```python
from build123d import *

# Parameters (mm, degrees)
BOSS_EXTRUDE1_DEPTH      = 54
BOSS_EXTRUDE1_DEPTH_BACK = 54
SKETCH2_R                = 18
SKETCH3_R                = 4
CUT_EXTRUDE1_DEPTH       = 122
SKETCH4_R                = 1.5
CUT_EXTRUDE2_DEPTH       = 5


with BuildPart() as part:
    # Sketch2 → Boss-Extrude1 (new, two sides: drawn at the far end of the back side and taken through both)
    with BuildSketch(Plane.XY.offset(-BOSS_EXTRUDE1_DEPTH_BACK)):
        Circle(SKETCH2_R)
    extrude(amount=BOSS_EXTRUDE1_DEPTH + BOSS_EXTRUDE1_DEPTH_BACK)

    # Sketch3 → Cut-Extrude1 (cut)
    with BuildSketch(Plane.XY.offset(54)):
        Circle(SKETCH3_R)
    extrude(amount=-CUT_EXTRUDE1_DEPTH, mode=Mode.SUBTRACT)

    # Sketch4 → Cut-Extrude2 (cut)
    with BuildSketch(Plane(origin=(0, 0, -54), x_dir=(-1, 0, 0), z_dir=(0, 0, -1))):
        with Locations((0, 14)):
            Circle(SKETCH4_R)
        with Locations((14, 0)):
            Circle(SKETCH4_R)
        with Locations((0, -14)):
            Circle(SKETCH4_R)
        with Locations((-14, 0)):
            Circle(SKETCH4_R)
    extrude(amount=-CUT_EXTRUDE2_DEPTH, mode=Mode.SUBTRACT)


solid = part.part
```
Could you check a few things on this model? Use its own coordinates, in mm. A direction names the side the tool comes from. Coordinates: 2 decimals unless noted, no trailing zeros. Order: outer loops, then holes, each group sorted by start corner. A loop starts at its lowest first (then second) coordinate and runs counter-clockwise, first axis right, second up. Notation, with made-up numbers: M 86,19 L 140,19 A21 ccw 140,46 Z; hole C -5.75,78.25 d9. An arc over 180 degrees is marked long. Use a Markdown table: item, result. Add a question column.
Q1. I want a section at A-A on y = 0. List the corners of the cut face in (x, z) for me, then the cut area to 3 significant figures.
Q2. We'd pull the mould along X, two halves only. Please class faces 1 (the cylindrical face through (-2.343, 17.847, -0.756)), 2 (the cylindrical face through (0.325, 12.536, -51.535)), 3 (the flat face through (-4.3, 0.3, 54)): pulls with the +X half, pulls with the -X half, needs draft (parallel to the pull), parting line crosses it, or undercut.
Q3. I want a section at C-C on z = 42. List the corners of the cut face in (x, y) for me, then the cut area to 3 significant figures.
Q4. I'm going to push flat-ended pins straight in: pin 1 (5 mm diameter, centred on x = -2, z = -30.5, fed in from +Y); pin 2 (4 mm diameter, centred on x = 13.5, z = -9, fed in from -Y); pin 3 (6 mm diameter, centred on x = 8.5, z = -30, fed in from +Y). Where does each tip first touch, or does it pass through?
Q5. If I drill on L1, parallel to Y at x = 0, z = -50; L2, parallel to Y at x = 0, z = -38; L3, parallel to Y at x = 3.5, z = 0.5, over which ranges is the centre line in solid material (lowest first)?
Q6. Which directions (+Z, -Z, +X, -X, +Y, -Y) give clear straight access to the entire face, cutting with the end or side of a thin tool? Please do faces 4 (the cylindrical face through (0.325, -15.464, -51.535)), 5 (the cylindrical face through (-0.867, -3.905, 0.756)).
Q7. I want a section at D-D on x = 14. List the corners of the cut face in (y, z) for me.
Checked values:
| question | item | result |
|---|---|---|
| 1 | outline | M -18,-54 L -15.5,-54 L -15.5,-49 L -12.5,-49 L -12.5,-54 L -4,-54 L -4,54 L -18,54 Z; M 4,-54 L 12.5,-54 L 12.5,-49 L 15.5,-49 L 15.5,-54 L 18,-54 L 18,54 L 4,54 Z |
| 1 | area | 2,990 mm² |
| 2 | face 1 | parting line crosses it |
| 2 | face 2 | undercut |
| 2 | face 3 | needs draft |
| 3 | outline | C 0,0 d36; hole C 0,0 d8 |
| 3 | area | 968 mm² |
| 4 | pin 1 | y = 18 |
| 4 | pin 2 | y = -13.85 |
| 4 | pin 3 | y = 17.14 |
| 5 | L1 | -18 to -15.5, -12.5 to -4, 4 to 12.5, 15.5 to 18 |
| 5 | L2 | -18 to -4, 4 to 18 |
| 5 | L3 | -17.66 to -1.94, 1.94 to 17.66 |
| 6 | face 4 | -Z |
| 6 | face 5 | +Z, -Z |
| 7 | outline | M -11.31,-54 L -1.5,-54 L -1.5,-49 L 1.5,-49 L 1.5,-54 L 11.31,-54 L 11.31,54 L -11.31,54 Z |
